Geometry: final body of the model. Coordinates: model frame, mm. A direction names the side the tool comes from. Round coordinates to 2 decimals unless told otherwise and drop trailing zeros. Loops run counter-clockwise (first coordinate to the right, second up) from the corner with the lowest first, then second, coordinate; pieces in that order, holes last. Notation, with made-up numbers: (3.25, 10) - (51.25, 10) arc R20 ccw to (51.25, 44) - close; hole circle Ø1 at (5, 58.25). An arc over 180 degrees is marked (long way). Answer as a JSON object with one key per item and string values. Group by question number.
Item 1: Section A-A (y = 0). Return the cut outline in (x, z), plus the area to 3 significant figures.
Item 2: Draft query along Z for faces 1 (the face through (20, -7, -9.95)), 2 (the face through (27, -28, 0)), 3 (the face through (0, -24, -17.5)). Return one class per face: released by +Z, released by -Z, zero draft, split by the parting line, or undercut.
Item 3: Section C-C (x = 0). Return the cut outline in (y, z).
Item 4: First-contact query: pin 1 (9 mm diameter, centred on y = -39, z = 5, fed in from +X); pin 2 (18.5 mm diameter, centred on x = 0, z = 0, fed in from -Y); pin 3 (12 mm diameter, centred on x = -19, z = 4.5, fed in from -Y); pin 4 (2 mm diameter, centred on x = 21, z = -3.5, fed in from -Y). Flat tips, straight axial feed; report the tip coordinate or a pass-through.
Item 5: Line query: line 1 (Z direction, x = -22, y = 4.5); line 2 (Y direction, x = 0, z = 13.75). Output: solid intervals per line, ascending.
Item 6: Section B-B (z = -13.5). Return the cut outline in (x, y), plus the area to 3 significant figures.
Item 7: Reachability of faces 4 (the face through (21, -30, 0)), 5 (the face through (20, -7, 9.95)), 6 (the face through (-27, 28, 0)), 7 (the face through (-17.5, -45, 0)), 8 (the face through (-30, 0, 0)) from +Z, -Z, +X, -X, +Y, -Y: full face, straight path, thin tool, end or side. Return the list, or none.
Item 8: Section D-D (x = 14). Return the cut outline in (y, z).
```python
from build123d import *

# Parameters (mm, degrees)
SKETCH_1_R          = 30
SKETCH_1_R_2        = 21
EXTRUDE_1_DEPTH     = 17.5
M22X1_5_1_D         = 20.5
M22X1_5_1_DEPTH     = 48.5
M22X1_5_1_TIP       = 6.158821345
CUT_EXTRUDE_START   = 8.25
SKETCH_5_R          = 22.75
SKETCH_5_R_2        = 21
CUT_EXTRUDE_1_DEPTH = 1.7
CHAMFER_1_SIZE      = 5


with BuildPart() as part:
    # 草图1 → 凸台-拉伸1 (new, symmetric)
    # profile 1 of 8: a face of its own
    with BuildSketch(Plane.XY):
        with BuildLine():
            Line((30, 30), (2.9e-08, 30))
            ThreePointArc((2.9e-08, 30), (21.213203446, 21.213203425), (30, 0))
            Line((30, 0), (30, 30))
        make_face()
    # profile 2 of 8: a face of its own
    with BuildSketch(Plane.XY):
        with BuildLine():
            Line((-30, 30), (-30, 0))
            ThreePointArc((-30, 0), (-21.213203425, 21.213203446), (2.9e-08, 30))
            Line((2.9e-08, 30), (-30, 30))
        make_face()
    # profile 3 of 8: a face of its own
    with BuildSketch(Plane.XY):
        Circle(SKETCH_1_R)
        Circle(SKETCH_1_R_2, mode=Mode.SUBTRACT)
    # profile 4 of 8: a face of its own
    with BuildSketch(Plane.XY):
        with BuildLine():
            Line((17.5, -24.366985862), (17.5, -30))
            Line((17.5, -30), (30, -30))
            Line((30, -30), (30, 0))
            ThreePointArc((30, 0), (26.69269563, -13.693063938), (17.5, -24.366985862))
        make_face()
    # profile 5 of 8: a face of its own
    with BuildSketch(Plane.XY):
        with BuildLine():
            ThreePointArc((17.5, -24.366985862), (9.192127723, -28.557044454), (0, -30))
            Line((0, -30), (17.5, -30))
            Line((17.5, -30), (17.5, -24.366985862))
        make_face()
    # profile 6 of 8: a face of its own
    with BuildSketch(Plane.XY):
        with BuildLine():
            ThreePointArc((0, -30), (-9.192127723, -28.557044454), (-17.5, -24.366985862))
            Line((-17.5, -24.366985862), (-17.5, -30))
            Line((-17.5, -30), (0, -30))
        make_face()
    # profile 7 of 8: a face of its own
    with BuildSketch(Plane.XY):
        with BuildLine():
            Line((-17.5, -30), (-17.5, -24.366985862))
            ThreePointArc((-17.5, -24.366985862), (-26.69269563, -13.693063938), (-30, 0))
            Line((-30, 0), (-30, -30))
            Line((-30, -30), (-17.5, -30))
        make_face()
    # profile 8 of 8: a face of its own
    with BuildSketch(Plane.XY):
        Polygon((0, -30), (-17.5, -30), (-17.5, -60), (17.5, -60), (17.5, -30), align=None)
    extrude(amount=EXTRUDE_1_DEPTH, both=True)

    # M22x1.5 螺纹孔1
    with Locations(Plane.XZ.offset(60)):
        with Locations((0, 0)):
            Hole(M22X1_5_1_D / 2, depth=M22X1_5_1_DEPTH)
            with Locations((0, 0, -(M22X1_5_1_DEPTH + M22X1_5_1_TIP / 2))):  # 118° drill point
                Cone(0, M22X1_5_1_D / 2, M22X1_5_1_TIP, mode=Mode.SUBTRACT)

    # 草图5 → 切除-拉伸1 (cut)
    with BuildSketch(Plane.XY.offset(CUT_EXTRUDE_START)):
        Circle(SKETCH_5_R)
        with Locations(Location((0, 0, 0), (0, 0, 253.16267609))):
            Circle(SKETCH_5_R_2, mode=Mode.SUBTRACT)
    cut_extrude_1 = extrude(amount=CUT_EXTRUDE_1_DEPTH, mode=Mode.SUBTRACT)

    # 镜向1: 切除-拉伸1 across plane
    add(cut_extrude_1.mirror(Plane.XY), mode=Mode.SUBTRACT)

    # 倒角1
    chamfer_1_edges = [part.edges().sort_by_distance(p)[0] for p in [
        (-30, -30, 0),
        (-30, 30, 0),
        (30, 30, 0),
        (30, -30, 0),
    ]]
    chamfer(chamfer_1_edges, length=CHAMFER_1_SIZE)


solid = part.part
```
Values:
{
 "1": {"outline": "(-30, -17.5) - (-21, -17.5) - (-21, -9.95) - (-22.75, -9.95) - (-22.75, -8.25) - (-21, -8.25) - (-21, 8.25) - (-22.75, 8.25) - (-22.75, 9.95) - (-21, 9.95) - (-21, 17.5) - (-30, 17.5) - close; (21, -17.5) - (30, -17.5) - (30, 17.5) - (21, 17.5) - (21, 9.95) - (22.75, 9.95) - (22.75, 8.25) - (21, 8.25) - (21, -8.25) - (22.75, -8.25) - (22.75, -9.95) - (21, -9.95) - close", "area": "618 mm^2"},
 "2": {"face 1": "undercut", "face 2": "zero draft", "face 3": "released by -Z"},
 "3": {"outline": "(-60, -17.5) - (-21, -17.5) - (-21, -10.25) - (-60, -10.25) - close; (-60, 10.25) - (-21, 10.25) - (-21, 17.5) - (-60, 17.5) - close; (21, -17.5) - (30, -17.5) - (30, 17.5) - (21, 17.5) - (21, 9.95) - (22.75, 9.95) - (22.75, 8.25) - (21, 8.25) - (21, -8.25) - (22.75, -8.25) - (22.75, -9.95) - (21, -9.95) - close"},
 "4": {"pin 1": "stops at x = 17.5", "pin 2": "stops at y = 18.85", "pin 3": "stops at y = -60", "pin 4": "stops at y = -30"},
 "5": {"line 1": "z = -17.5 to -9.95, -8.25 to 8.25, 9.95 to 17.5", "line 2": "y = -60 to -21, 21 to 30"},
 "6": {"outline": "(-30, -25) - (-25, -30) - (-17.5, -30) - (-17.5, -60) - (17.5, -60) - (17.5, -30) - (25, -30) - (30, -25) - (30, 25) - (25, 30) - (-25, 30) - (-30, 25) - close; hole circle Ø42 at (0, 0)", "area": "3,210 mm^2"},
 "7": {"face 4": "+Z, -Z, +X, -Y", "face 5": "none", "face 6": "+Z, -Z, -X, +Y", "face 7": "+Z, -Z, -X, -Y", "face 8": "+Z, -Z, -X, +Y, -Y"},
 "8": {"outline": "(-60, -17.5) - (-15.65, -17.5) - (-15.65, -9.95) - (-17.93, -9.95) - (-17.93, -8.25) - (-15.65, -8.25) - (-15.65, 8.25) - (-17.93, 8.25) - (-17.93, 9.95) - (-15.65, 9.95) - (-15.65, 17.5) - (-60, 17.5) - close; (15.65, -17.5) - (30, -17.5) - (30, 17.5) - (15.65, 17.5) - (15.65, 9.95) - (17.93, 9.95) - (17.93, 8.25) - (15.65, 8.25) - (15.65, -8.25) - (17.93, -8.25) - (17.93, -9.95) - (15.65, -9.95) - close"}
}
